For this review, take the finished solid that the model builds, in its own axes (mm). Round coordinates to 2 decimals unless told otherwise and drop trailing zeros. Loops run counter-clockwise (first coordinate to the right, second up) from the corner with the lowest first, then second, coordinate; pieces in that order, holes last. Notation, with made-up numbers: M 45,38.5 L 62,38.5 A23 cw 62,51.5 Z; hole C 89,70 d4. An arc over 180 degrees is marked long. One line per question, with ' | ' between items. Start each with the question number.
1) For probe 1 along Z at (x, y) = (7.75, 103.5); probe 2 along Z at (x, y) = (7.5, 98); probe 3 along Y at (x, z) = (11.25, 330.5), list the stretches that pass through material, from the lowest coordinate up. Write a range as from..to.
2) We need section A-A (x = 5.75). Give the boundary of the cut face in (y, z).
3) Mouldability with a two-part tool opening along Y and no side actions: class faces 1 (the face through (6, 50.548, 207)), 2 (the face through (6.439, 98.837, 305.508)), 3 (the face through (6.44, 148.33, 69.59)) as pulls with the +Y half, pulls with the -Y half, needs draft (parallel to the pull), parting line crosses it, or undercut.
Autodesk Inventor part; units mm, degrees
ref_plane "YZ Plane" through (0, 0, 0) normal (1, 0, 0) x (0, 1, 0)
ref_plane "XZ Plane" through (0, 0, 0) normal (0, 1, 0) x (-1, 0, 0)
ref_plane "XY Plane" through (0, 0, 0) normal (0, 0, 1) x (1, 0, 0)
sketch "Sketch1" plane through (0, 0, 0) normal (1, 0, 0) x (0, 1, 0)
  line L0 (152.1482, 345.366) -> (50.5482, 345.366)
  line L1 (50.5482, 345.366) -> (50.5482, 65.966)
  line L2 (50.5482, 65.966) -> (152.1482, 65.966)
  line L3 (152.1482, 65.966) -> (152.1482, 345.366)
  point P0 (0, 0)
  dimension "d0" = 279.4
  dimension "d1" = 101.6
extrude "Extrusion1" add sketch "Sketch1" along normal blind 12.7
fillet "Fillet1" radius 12.7 4 edges at (6.35, 152.1482, 345.366) (6.35, 152.1482, 65.966) (6.35, 50.5482, 345.366) (6.35, 50.5482, 65.966)
sketch "Sketch2" plane through (12.7, 0, 0) normal (1, 0, 0) x (0, 0, -1)
  line L0 (-345.366, 139.4482) -> (-345.366, 63.2482)
  line L1 (-345.366, 101.3482) -> (-65.966, 101.3482)
  line L2 (-65.966, 63.2482) -> (-65.966, 139.4482)
  line L3 (-345.366, 152.1482) -> (-334.254, 152.0486)
  arc A0 (-332.666, 152.1482) -> (-345.366, 139.4482) centre (-332.666, 139.4482) ccw
  line L4 (-334.254, 152.0486) -> (-334.254, 101.3482)
  circle A1 centre (-334.254, 101.3482) radius 6.35
  point P0 (0, 0)
  dimension "d5" = 11.1125
  dimension "d6" = 12.7
extrude "Extrusion2" cut sketch "Sketch2" against normal blind 42.8625 contours A1 L4 L1 | L1 A1 | A1 L1 L4
sketch "Sketch3" plane through (12.7, 0, 0) normal (1, 0, 0) x (0, 0, -1)
  line L0 (-345.366, 152.1482) -> (-307.266, 152.1482)
  line L1 (-78.666, 152.1482) -> (-332.666, 152.1482)
  line L2 (-307.266, 152.1482) -> (-307.266, 102.2169)
  circle A0 centre (-307.266, 102.2169) radius 3.81
  point P0 (0, 0)
  dimension "d9" = 38.1
  dimension "d10" = 7.62
extrude "Extrusion3" cut sketch "Sketch3" against normal blind 88.9
sketch "Sketch4" plane through (12.7, 0, 0) normal (1, 0, 0) x (0, 0, -1)
  line L0 (-65.966, 63.2482) -> (-65.966, 139.4482)
  line L1 (-65.966, 103.1393) -> (-299.4746, 103.1393)
  point P0 (0, 0)
sketch "Sketch5" plane through (12.7, 0, 0) normal (1, 0, 0) x (0, 0, -1)
  line L0 (-345.366, 152.1482) -> (-205.666, 152.1482)
  line L1 (-78.666, 152.1482) -> (-332.666, 152.1482)
  line L2 (-205.666, 103.8134) -> (-205.666, 152.1482)
  circle A0 centre (-205.666, 103.8134) radius 3.81
  point P0 (0, 0)
  dimension "d13" = 7.62
extrude "Extrusion4" cut sketch "Sketch5" against normal blind 214.3125
sketch "Sketch6" plane through (12.7, 0, 0) normal (1, 0, 0) x (0, 0, -1)
  line L0 (-65.966, 152.1482) -> (-77.0785, 152.1482)
  line L1 (-78.666, 152.1482) -> (-332.666, 152.1482)
  line L2 (-77.0785, 152.1482) -> (-77.0785, 103.1012)
  circle A0 centre (-77.0785, 103.1012) radius 6.35
  point P0 (0, 0)
  dimension "d16" = 11.1125
  dimension "d17" = 12.7
extrude "Extrusion5" cut sketch "Sketch6" against normal blind 211.1375
sketch "Sketch7" plane through (12.7, 0, 0) normal (1, 0, 0) x (0, 0, -1)
  point P0 (0, 0)
properties part number "Base Plate."
Answers below:
1) probe 1: 65.97..70.74, 83.42..201.87, 209.46..303.68, 310.85..328.28, 340.23..345.37 | probe 2: 65.97..73.3, 80.86..328.86, 339.65..345.37 | probe 3: 50.55..96.23, 106.47..152.15
2) outline: M 50.55,78.67 A12.7 ccw 63.25,65.97 L 139.45,65.97 A12.7 ccw 152.15,78.67 L 152.15,332.67 A12.7 ccw 139.45,345.37 L 63.25,345.37 A12.7 ccw 50.55,332.67 Z; hole C 101.35,334.25 d12.7; hole C 103.1,77.08 d12.7; hole C 102.22,307.27 d7.62; hole C 103.81,205.67 d7.62
3) face 1: pulls with the -Y half | face 2: undercut | face 3: pulls with the +Y half
